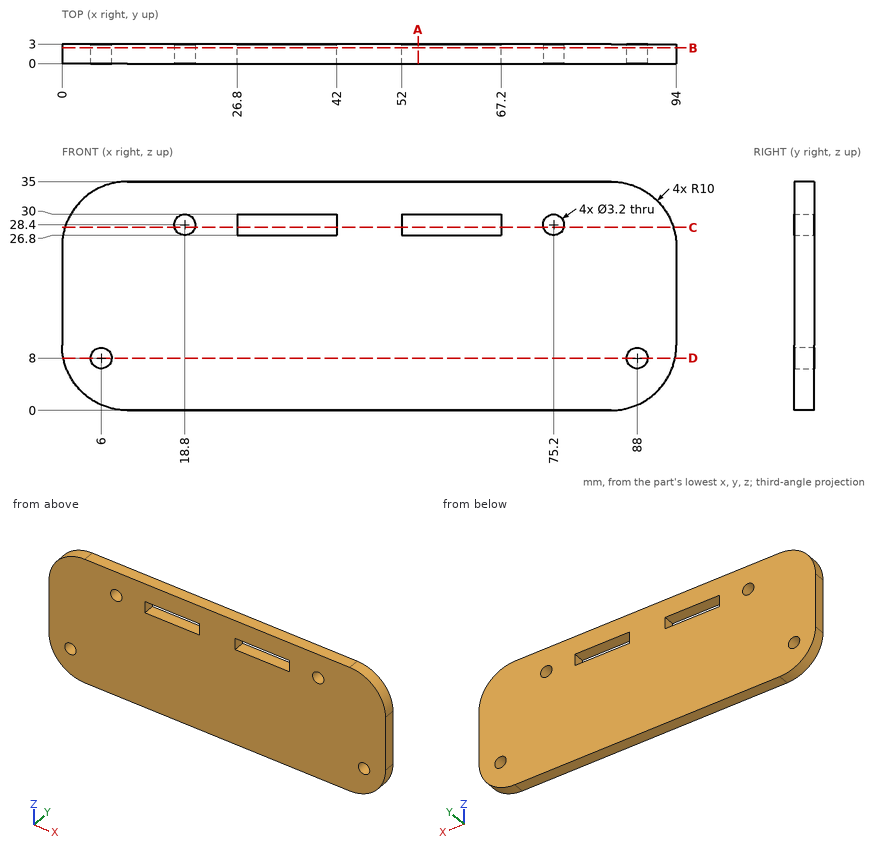
Study the drawing (mm; zero at the part's minimum x, y, z) and answer. Round coordinates to 2 decimals unless told otherwise and drop trailing zeros. Write each loop counter-clockwise with the first axis right and the second up, starting at its lowest first coordinate (ties: lowest second). Pieces come first, ordered by that corner, then holes. Notation, with made-up numbers: (22, -18.5) -> (49, -18.5) arc R19 cw to (49, -12.5) -> close; hole circle Ø9 at (61.5, 24.5). An arc over 180 degrees is marked (long way). Write item = value, one per line.
1) Section D-D on z = 8 is taken. Write down the section's boundary in (x, y), plus the area to 3 significant figures.
Check values:
outline = (0.2, 0) -> (4.4, 0) -> (4.4, 3) -> (0.2, 3) -> close; (7.6, 0) -> (86.4, 0) -> (86.4, 3) -> (7.6, 3) -> close; (89.6, 0) -> (93.8, 0) -> (93.8, 3) -> (89.6, 3) -> close
area = 262 mm²
2) Section C-C on z = 28 is taken. Write down the section's boundary in (x, y), plus the area to 3 significant figures.
Check values:
outline = (0.46, 0) -> (17.25, 0) -> (17.25, 3) -> (0.46, 3) -> close; (20.35, 0) -> (26.8, 0) -> (26.8, 3) -> (20.35, 3) -> close; (42, 0) -> (52, 0) -> (52, 3) -> (42, 3) -> close; (67.2, 0) -> (73.65, 0) -> (73.65, 3) -> (67.2, 3) -> close; (76.75, 0) -> (93.54, 0) -> (93.54, 3) -> (76.75, 3) -> close
area = 169 mm²
3) Straight lines are drawn through the part: line 1 along X through (y, z) = (2, 8); line 2 along X through (y, z) = (1.3, 28.4); line 3 along Z through (x, y) = (35, 0.3). For each, find the intervals that lie inside material, in ascending order. Write a range as [from, to].
Check values:
line_1 = [0.2, 4.4], [7.6, 86.4], [89.6, 93.8]
line_2 = [0.6, 17.2], [20.4, 26.8], [42, 52], [67.2, 73.6], [76.8, 93.4]
line_3 = [0, 26.8], [30, 35]
4) Section A-A on x = 54.5 is taken. Write down the section's boundary in (y, z), plus the area to 3 significant figures.
Check values:
outline = (0, 0) -> (3, 0) -> (3, 26.8) -> (0, 26.8) -> close; (0, 30) -> (3, 30) -> (3, 35) -> (0, 35) -> close
area = 95.4 mm²
5) Section B-B on y = 2.4 is taken. Write down the section's boundary in (x, z), plus the area to 3 significant figures.
Check values:
outline = (0, 10) arc R10 ccw to (10, 0) -> (84, 0) arc R10 ccw to (94, 10) -> (94, 25) arc R10 ccw to (84, 35) -> (10, 35) arc R10 ccw to (0, 25) -> close; hole circle Ø3.2 at (6, 8); hole circle Ø3.2 at (18.8, 28.4); hole (26.8, 26.8) -> (42, 26.8) -> (42, 30) -> (26.8, 30) -> close; hole (52, 26.8) -> (67.2, 26.8) -> (67.2, 30) -> (52, 30) -> close; hole circle Ø3.2 at (75.2, 28.4); hole circle Ø3.2 at (88, 8)
area = 3,070 mm²
6) Given pin 1 (1.5 mm diameter, centred on x = 36.5, y = 2, fed in from -Z); pin 2 (1.5 mm diameter, centred on y = 2, z = 28, fed in from -X); pin 3 (1.5 mm diameter, centred on y = 2, z = 29, fed in from +X), each flat-ended and moving along its own axis, determine where each tip first touches the part or whether it passes through.
Check values:
pin_1 = 0
pin_2 = 0.26
pin_3 = 93.46
